Design review of the part built by this model. Coordinates are the model's own, in mm. A direction names the side the tool comes from. Coordinates: 2 decimals unless noted, no trailing zeros. Loops run counter-clockwise (first coordinate to the right, second up) from the corner with the lowest first, then second, coordinate; pieces in that order, holes last. Notation, with made-up numbers: M -31,16.5 L 26,16.5 A8 cw 26,24.5 Z; hole C 64.5,15.25 d1. An arc over 180 degrees is marked long. Answer as CSV lines item,"result". Start each with the question number.
from build123d import *

# Parameters (mm, degrees)
ESBO_O1_W                = 70
ESBO_O1_H                = 40
ESBO_O1_R                = 3.97
RESSALTO_EXTRUS_O1_DEPTH = 15
ESBO_O3_R                = 3.97
CORTE_EXTRUS_O2_DEPTH    = 15
ESBO_O4_R                = 3.97
CORTE_EXTRUS_O3_DEPTH    = 20
CHANFRO2_SIZE            = 7


with BuildPart() as part:
    # Esboço1 → Ressalto-extrusão1 (new body, symmetric)
    with BuildSketch(Plane(origin=(0, 0, 0), x_dir=(0, 0, -1), z_dir=(1, 0, 0))):
        Rectangle(ESBO_O1_W, ESBO_O1_H)
        with Locations((-20, 0)):
            Circle(ESBO_O1_R, mode=Mode.SUBTRACT)
        with Locations((20, 0)):
            Circle(ESBO_O1_R, mode=Mode.SUBTRACT)
    extrude(amount=RESSALTO_EXTRUS_O1_DEPTH, both=True)

    # Esboço3 → Corte-extrusão2 (cut)
    with BuildSketch(Plane.XY.offset(35)):
        Circle(ESBO_O3_R)
    extrude(amount=-CORTE_EXTRUS_O2_DEPTH, mode=Mode.SUBTRACT)

    # Esboço4 → Corte-extrusão3 (cut)
    with BuildSketch(Plane(origin=(0, 20, 0), x_dir=(1, 0, 0), z_dir=(0, 1, 0))):
        with Locations((0, 20)):
            Circle(ESBO_O4_R)
        with Locations((0, -20)):
            Circle(ESBO_O4_R)
    extrude(amount=-CORTE_EXTRUS_O3_DEPTH, mode=Mode.SUBTRACT)

    # Chanfro2
    chanfro2_edges = [part.edges().sort_by_distance(p)[0] for p in [
        (0, 20, 35),
        (0, 20, -35),
    ]]
    chamfer(chanfro2_edges, length=CHANFRO2_SIZE)


solid = part.part
Item 1: For faces 4 (the face through (-0.861, -3.876, 29.272)), 5 (the face through (0, 17, 31)), 6 (the face through (-3.966, 12.362, -20.175)), list the 3-axis set-ups (+Z, -Z, +X, -X, +Y, -Y) from which the entire face can be reached by the end or side of a thin tool; tool diameter is ignored.
Item 2: Add section B-B (x = 0). Give the boundary of the cut face in (y, z).
Item 3: Add section C-C (y = 10.5). Give the boundary of the cut face in (x, z).
Item 4: Add section A-A (z = -20). Give the boundary of the cut face in (x, y).
Item 5: Add section D-D (x = 6.5). Give the boundary of the cut face in (y, z).
Item 6: For pin 1 (9 mm diameter, centred on y = 0, z = -20, fed in from -X), flat-tipped, find the tip position at first contact; note if it passes through.
Item 7: Mouldability with a two-part tool opening along Z and no side actions: class faces 1 (the face through (-15, 0, 0)), 2 (the face through (-0.21, -1.521, 16.333)), 3 (the face through (0, -4, -35)) as released by +Z, released by -Z, zero draft, split by the parting line, or undercut.
Item 8: For line 1 along Z through (x, y) = (0, 11.25); line 2 along Z through (x, y) = (-6.5, 3.5); line 3 along X through (y, z) = (7.75, 20), list the stretches that pass through material, from the lowest coordinate up. Write a range as from..to.
Response:
1,face 4,"+Z"
1,face 5,"+Z, +X, -X, +Y"
1,face 6,"+Y"
2,outline,"M -20,-35 L 13,-35 L 20,-28 L 20,-23.97 L 0,-23.97 A3.97 cw 0,-16.03 L 20,-16.03 L 20,16.03 L 0,16.03 A3.97 cw -3.97,20 L -3.97,35 L -20,35 Z; M 3.97,23.97 L 20,23.97 L 20,28 L 13,35 L 3.97,35 Z"
3,outline,"M -15,-35 L 15,-35 L 15,35 L -15,35 Z; hole C 0,-20 d7.94; hole C 0,20 d7.94"
4,outline,"M -15,-20 L 15,-20 L 15,-3.97 L -15,-3.97 Z; M -15,3.97 L -3.97,3.97 L -3.97,20 L -15,20 Z; M 3.97,3.97 L 15,3.97 L 15,20 L 3.97,20 Z"
5,outline,"M -20,-35 L 13,-35 L 20,-28 L 20,28 L 13,35 L -20,35 Z; hole C 0,-20 d7.94; hole C 0,20 d7.94"
6,pin 1,"x = -15"
7,face 1,"zero draft"
7,face 2,"undercut"
7,face 3,"released by -Z"
8,line 1,"-35..-23.97, -16.03..16.03, 23.97..35"
8,line 2,"-35..-21.87, -18.13..18.13, 21.87..35"
8,line 3,"-15..-3.97, 3.97..15"
